from build123d import *

# Parameters (mm, degrees)
SKETCH1_R                       = 11
BOSS_EXTRUDE1_DEPTH             = 57.2
TAP_DRILL_FOR_M2X0_4_TAP1_D     = 1.6
TAP_DRILL_FOR_M2X0_4_TAP1_DEPTH = 4
TAP_DRILL_FOR_M2X0_4_TAP1_TIP   = 0.480688495
BOSS_EXTRUDE2_DEPTH             = 2.5
BOSS_EXTRUDE3_DEPTH             = 15.3


with BuildPart() as part:
    # Sketch1 → Boss-Extrude1 (new body)
    with BuildSketch(Plane(origin=(0, 0, 0), x_dir=(0, 0, -1), z_dir=(1, 0, 0))):
        Circle(SKETCH1_R)
    extrude(amount=BOSS_EXTRUDE1_DEPTH)

    # Tap Drill for M2x0.4 Tap1
    with Locations(Plane(origin=(57.2, 0, 0), x_dir=(0, 0, -1), z_dir=(1, 0, 0))):
        with Locations((9, 0), (0, 9), (-9, 0), (0, -9)):
            Hole(TAP_DRILL_FOR_M2X0_4_TAP1_D / 2, depth=TAP_DRILL_FOR_M2X0_4_TAP1_DEPTH)
            with Locations((0, 0, -(TAP_DRILL_FOR_M2X0_4_TAP1_DEPTH + TAP_DRILL_FOR_M2X0_4_TAP1_TIP / 2))):  # 118° drill point
                Cone(0, TAP_DRILL_FOR_M2X0_4_TAP1_D / 2, TAP_DRILL_FOR_M2X0_4_TAP1_TIP, mode=Mode.SUBTRACT)

    # Sketch4 → Boss-Extrude2 (add)
    with BuildSketch(Plane(origin=(57.2, 0, 0), x_dir=(0, 0, -1), z_dir=(1, 0, 0))):
        with BuildLine():
            Line((4.877567481, -4.296432877), (4.877567481, 4.296432877))
            ThreePointArc((4.877567481, 4.296432877), (0, 6.5), (-4.877567481, 4.296432877))
            Line((-4.877567481, 4.296432877), (-4.877567481, -4.296432877))
            ThreePointArc((-4.877567481, -4.296432877), (0, -6.5), (4.877567481, -4.296432877))
        make_face()
    extrude(amount=BOSS_EXTRUDE2_DEPTH)

    # Sketch5 → Boss-Extrude3 (add)
    with BuildSketch(Plane(origin=(59.7, 0, 0), x_dir=(0, 0, -1), z_dir=(1, 0, 0))):
        with BuildLine():
            Line((1.765106223, -0.940425447), (1.765106223, 0.940425447))
            ThreePointArc((1.765106223, 0.940425447), (-2, 0), (1.765106223, -0.940425447))
        make_face()
    extrude(amount=BOSS_EXTRUDE3_DEPTH)


solid = part.part
Read the model definition and answer for the solid it produces. Units are mm, in the model's axes. A direction names the side the tool comes from. Coordinates: 2 decimals unless noted, no trailing zeros. Order: outer loops, then holes, each group sorted by start corner. A loop starts at its lowest first (then second) coordinate and runs counter-clockwise, first axis right, second up. Notation, with made-up numbers: (-39, 44) -> (8, 44) arc R35 cw to (8, 79) -> close; hole circle Ø7 at (-13, 84). An arc over 180 degrees is marked (long way). Answer as a JSON object with one key per item and string values.
1) Each of these flat-tipped pins is pushed along its axis until it touches: pin 1 (1 mm diameter, centred on y = -9, z = 0, fed in from +X); pin 2 (4 mm diameter, centred on x = 33, z = 5, fed in from -Y); pin 3 (1.4 mm diameter, centred on y = 9, z = 0, fed in from +X). Where does it stop, or does it pass through?
Model answer:
{"pin 1": "stops at x = 53.02", "pin 2": "stops at y = -10.58", "pin 3": "stops at x = 53.14"}
2) Consider line 1 along Y through (x, z) = (55.2, 0); line 2 along X through (y, z) = (-6.5, -4.5); line 3 along X through (y, z) = (-3, 1.75). Determine where each line is inside the solid, lowest interval first. Write a range as from..to.
Model answer:
{"line 1": "y = -11..-9.8, -8.2..8.2, 9.8..11", "line 2": "x = 0..57.2", "line 3": "x = 0..59.7"}
3) A tool of negligible diameter and unlimited length cuts with its end or side. For faces 1 (the face through (55.2, 0, -9.8)), 2 (the face through (58, 0, 4.878)), 3 (the face through (58, 0, -4.878)), 4 (the face through (58.4, 6.5, -0.1)), from which of +Z, -Z, +X, -X, +Y, -Y can it reach the whole face along a straight path? Write none if from no direction.
Model answer:
{"face 1": "+X", "face 2": "+Z, +X, +Y, -Y", "face 3": "-Z, +X, +Y, -Y", "face 4": "+X, +Y"}
4) A cutting plane is placed at A-A, the plane x = 68.5. Determine the outline of the cut face in (y, z), plus the area to 3 significant figures.
Model answer:
{"outline": "(-0.94, -1.77) -> (0.94, -1.77) arc R2 ccw (long way) to start", "area": "12.3 mm²"}
5) A cutting plane is placed at C-C, the plane x = 6.5. Determine the outline of the cut face in (y, z).
Model answer:
{"outline": "circle Ø22 at (0, 0)"}
6) The mould has two halves that part along Z. Classify faces 5 (the face through (58.4, -6.5, 0.1)), 6 (the face through (52.803, 9.138, 0.018)), 7 (the face through (67, 0, -1.765)), 8 (the face through (52.803, 0.006, 9.139)): released by +Z, released by -Z, zero draft, split by the parting line, or undercut.
Model answer:
{"face 5": "split by the parting line", "face 6": "undercut", "face 7": "released by -Z", "face 8": "undercut"}
7) A cutting plane is placed at B-B, the plane z = 6. Determine the outline of the cut face in (x, y), plus the area to 3 significant figures.
Model answer:
{"outline": "(0, -9.22) -> (57.2, -9.22) -> (57.2, 9.22) -> (0, 9.22) -> close", "area": "1,050 mm²"}
